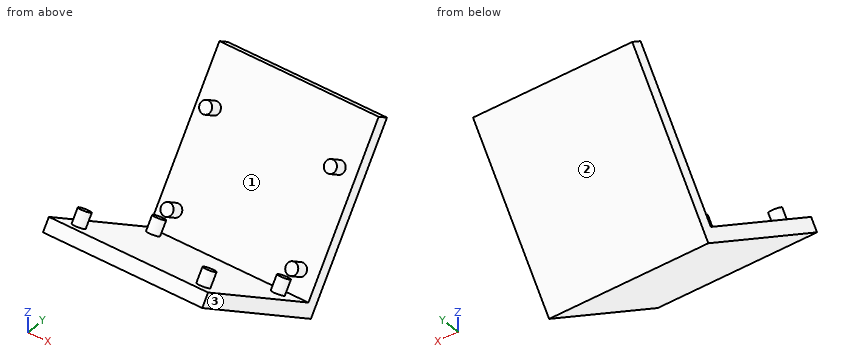
```python
from build123d import *

# Parameters (mm, degrees)
PAD008_DEPTH            = 60
SKETCH028_R             = 4.5
PAD009_DEPTH            = 10.5
SKETCH026_R             = 4.5
PAD010_DEPTH            = 10.5
BODY005_PLACEMENT_ANGLE = 145


with BuildPart() as part:
    # Sketch027 → Pad008 (new body, symmetric)
    with BuildSketch(Plane.YZ):
        Polygon((-10, 10), (-10, -110), (-20, -110), (-20, 20), (110, 20), (110, 10), align=None)
    extrude(amount=PAD008_DEPTH, both=True)

    # Sketch028 → Pad009 (join)
    with BuildSketch(Plane(origin=(0, -10, 0), x_dir=(-1, 0, 0), z_dir=(0, 1, 0))):
        with Locations((-47, -6)):
            Circle(SKETCH028_R)
        with Locations((-47, -72)):
            Circle(SKETCH028_R)
        with Locations((47, -6)):
            Circle(SKETCH028_R)
        with Locations((47, -72)):
            Circle(SKETCH028_R)
    extrude(amount=PAD009_DEPTH)

    # Sketch026 → Pad010 (join)
    with BuildSketch(Plane(origin=(0, 0, 10), x_dir=(-1, 0, 0), z_dir=(0, 0, -1))):
        with Locations((-47, 6)):
            Circle(SKETCH026_R)
        with Locations((-47, 95)):
            Circle(SKETCH026_R)
        with Locations((47, 95)):
            Circle(SKETCH026_R)
        with Locations((47, 6)):
            Circle(SKETCH026_R)
    extrude(amount=PAD010_DEPTH)


with BuildPart() as part_1:
    # Body005 placement: moved
    add(part.part.moved(Location((0, 19.28038, -55.844471))).rotate(Axis((0, 19.28038, -55.844471), (1, 0, 0)), BODY005_PLACEMENT_ANGLE))


solid = part_1.part
```
For this review, take the finished solid that the model builds, in its own axes (mm). Face numbers are marked on the shaded views. Give positions to 0.01 mm unless a question says otherwise; leave off trailing zeros. Write each loop counter-clockwise with the first axis right and the second up, starting at its lowest first coordinate (ties: lowest second). Pieces come first, ordered by that corner, then holes. Notation, with made-up numbers: M -13,39.25 L 20,39.25 A13 cw 20,51.25 Z; hole C 18.5,8.25 d6. An arc over 180 degrees is marked long. Answer as CSV lines item,"result".
1. Consider section A-A, the plane z = -32. Write out the cut boundary in (x, y).
Findings:
outline,"M -60,-49.64 L 60,-49.64 L 60,-32.21 L -60,-32.21 Z; M -60,48.18 L 60,48.18 L 60,60.39 L -60,60.39 Z"
2. Draft analysis for pull direction Y (two halves, no side actions). For the marked faces 1, 2 and 3, state which applies: +Y half, -Y half, draft (parallel to the pull), parting line (faces both ways), or undercut.
Findings:
face 1,"undercut"
face 2,"+Y half"
face 3,"draft"
3. For pin 1 (12 mm diameter, centred on x = -15.5, z = 1.5, fed in from +Y); pin 2 (3 mm diameter, centred on x = 37, z = 8, fed in from -Y); pin 3 (1.5 mm diameter, centred on x = 28, z = -30, fed in from +Y), all flat-tipped, find the tip position at first contact; note any pin that passes through.
Findings:
pin 1,"stops at y = 88.05"
pin 2,"stops at y = 75.14"
pin 3,"stops at y = 62.32"
4. Consider section D-D, the plane z = 19. Write out the cut boundary in (x, y).
Findings:
outline,"M -60,83.89 L 60,83.89 L 60,96.1 L -60,96.1 Z"
5. Wall thickness on line 1 (Y direction, x = -49, z = -40); line 2 (Y direction, x = -52, z = -13.5); line 3 (X direction, y = 26, z = -51.5): over which ranges is each line inside the solid? List them lowest first.
Findings:
line 1,"y = -38.22 to -20.78, 42.58 to 54.79"
line 2,"y = -76.06 to -58.63, 61.14 to 73.35"
line 3,"x = -51.27 to -42.73, 42.73 to 51.27"
6. Consider section C-C, the plane y = -28. Write out the cut boundary in (x, z).
Findings:
outline,"M -60,-47.15 L 60,-47.15 L 60,-34.95 L -60,-34.95 Z"
7. Consider section B-B, the plane x = -11.5. Write out the cut boundary in (y, z).
Findings:
outline,"M -82.3,-9.13 L 24.19,-83.7 L 98.76,22.79 L 90.57,28.53 L 21.74,-69.77 L -76.56,-0.94 Z"
